```python
from build123d import *
from OCP.BRepFilletAPI import BRepFilletAPI_MakeChamfer

# Parameters (mm, degrees)
SKETCH1_W           = 76.2
SKETCH1_H           = 76.2
SKETCH1_W_2         = 69.85
SKETCH1_H_2         = 69.85
BOSS_EXTRUDE1_DEPTH = 9.525
SKETCH2_R           = 1.26365
CUT_EXTRUDE1_DEPTH  = 86.725
CHAMFER1_SIZE       = 2.54
CHAMFER1_SIZE2      = 2.207988314
SKETCH3_W           = 76.2
SKETCH3_H           = 76.2
SKETCH3_W_2         = 69.85
SKETCH3_H_2         = 69.85
BOSS_EXTRUDE2_DEPTH = 25.4


with BuildPart() as part:
    # Sketch1 → Boss-Extrude1 (new body)
    with BuildSketch(Plane(origin=(0, 0, 0), x_dir=(1, 0, 0), z_dir=(0, 1, 0))):
        Rectangle(SKETCH1_W, SKETCH1_H)
        Rectangle(SKETCH1_W_2, SKETCH1_H_2, mode=Mode.SUBTRACT)
    extrude(amount=BOSS_EXTRUDE1_DEPTH)

    # Sketch2 → Cut-Extrude1 (cut, through all)
    with BuildSketch(Plane.XY.offset(38.1)):
        with Locations((-12.7, 4.7625)):
            Circle(SKETCH2_R)
        with Locations((12.7, 4.7625)):
            Circle(SKETCH2_R)
    extrude(amount=-CUT_EXTRUDE1_DEPTH, mode=Mode.SUBTRACT)

    # Chamfer1: one chamfer whose edges measure the first distance from different faces: ONE call of the kernel's chamfer builder (chamfer() names one face for all edges)
    chamfer1_edges_1 = [part.edges().sort_by_distance(p)[0] for p in [
        (-13.96365, 4.7625, -38.1),
    ]]
    chamfer1_side_1 = [part.faces().sort_by_distance(p)[0] for p in [
        (-13.96365, 4.7625, -36.5125),
    ]]
    chamfer1_edges_2 = [part.edges().sort_by_distance(p)[0] for p in [
        (-13.96365, 4.7625, 38.1),
        (11.43635, 4.7625, 38.1),
    ]]
    chamfer1_side_2 = [part.faces().sort_by_distance(p)[0] for p in [
        (0, 4.7625, 38.1),
    ]]
    chamfer1_edges_3 = [part.edges().sort_by_distance(p)[0] for p in [
        (11.43635, 4.7625, -38.1),
    ]]
    chamfer1_side_3 = [part.faces().sort_by_distance(p)[0] for p in [
        (11.43635, 4.7625, -36.5125),
    ]]
    chamfer1 = BRepFilletAPI_MakeChamfer(part.part.solid().wrapped)
    for e in chamfer1_edges_1:
        chamfer1.Add(CHAMFER1_SIZE, CHAMFER1_SIZE2, e.wrapped, chamfer1_side_1[0].wrapped)  # the first distance lies on this face
    for e in chamfer1_edges_2:
        chamfer1.Add(CHAMFER1_SIZE, CHAMFER1_SIZE2, e.wrapped, chamfer1_side_2[0].wrapped)  # the first distance lies on this face
    for e in chamfer1_edges_3:
        chamfer1.Add(CHAMFER1_SIZE, CHAMFER1_SIZE2, e.wrapped, chamfer1_side_3[0].wrapped)  # the first distance lies on this face
    add(Compound.cast(chamfer1.Shape()), mode=Mode.REPLACE)

    # Sketch3 → Boss-Extrude2 (add)
    with BuildSketch(Plane(origin=(0, 9.525, 0), x_dir=(1, 0, 0), z_dir=(0, 1, 0))):
        Rectangle(SKETCH3_W, SKETCH3_H)
        Rectangle(SKETCH3_W_2, SKETCH3_H_2, mode=Mode.SUBTRACT)
    extrude(amount=BOSS_EXTRUDE2_DEPTH)

    # Mirror2: part across plane


with BuildPart() as part_1:
    add(part.part)
    add(part.part.mirror(Plane.ZX.offset(34.925)))


solid = part_1.part
```
Work out the finished part from the listing and answer in its coordinate system (mm). A direction names the side the tool comes from. Give positions to 0.01 mm unless a question says otherwise; leave off trailing zeros. Order: outer loops, then holes, each group sorted by start corner. A loop starts at its lowest first (then second) coordinate and runs counter-clockwise, first axis right, second up.
1. Section C-C, the plane x = 12.7 is taken. Give the number of separate pieces and of enclosed holes in the cut face, and give its area (3 significant figures).
Result sheet:
separate pieces: 6
enclosed holes: 0
area: 389 mm2
2. Straight lines are drawn through the part: L1, parallel to Y at x = 12.7, z = -35.3; L2, parallel to X at y = 38, z = 26.5 (3 decimals). For each, find the intervals that lie inside material, in ascending order.
Result sheet:
L1: y = 0 to 3.5, 6.03 to 63.82, 66.35 to 69.85
L2: x = -38.1 to -34.925, 34.925 to 38.1
3. Section B-B, the plane y = 51 is taken. Determine the outline of the cut face in (x, z) (3 decimals).
Result sheet:
outline: (-38.1, -38.1) - (38.1, -38.1) - (38.1, 38.1) - (-38.1, 38.1) - close; hole (-34.925, -34.925) - (34.925, -34.925) - (34.925, 34.925) - (-34.925, 34.925) - close
4. Section A-A, the plane x = -3 is taken. Determine the outline of the cut face in (y, z) (3 decimals).
Result sheet:
outline: (0, -38.1) - (69.85, -38.1) - (69.85, -34.925) - (0, -34.925) - close; (0, 34.925) - (69.85, 34.925) - (69.85, 38.1) - (0, 38.1) - close
5. The mould has two halves that part along Z. Classify faces 3 (the flat face through (0, 35, 34.925)), 4 (the flat face through (-1, 35, 38.1)), 5 (the flat face through (-1, 35, -38.1)): released by +Z, released by -Z, zero draft, split by the parting line, or undercut.
Result sheet:
face 3: undercut
face 4: released by +Z
face 5: released by -Z
6. Each of these flat-tipped pins is pushed along its axis until it touches: P1, Ø3, axis at x = 12.7, y = 65.09, coming from the -Z side; P2, Ø3.5, axis at x = -12.7, y = 4.76, coming from the -Z side; P3, Ø4, axis at x = 12.7, y = 65.09, coming from the -Z side. Where does it stop, or does it pass through?
Result sheet:
P1: stops at z = -35.83
P2: stops at z = -36.12
P3: stops at z = -36.41
7. Section D-D, the plane z = -14.5 is taken. Determine the outline of the cut face in (x, y) (3 decimals).
Result sheet:
outline: (-38.1, 0) - (-34.925, 0) - (-34.925, 69.85) - (-38.1, 69.85) - close; (34.925, 0) - (38.1, 0) - (38.1, 69.85) - (34.925, 69.85) - close
8. For faces 1 (the flat face through (-34.925, 35, 0)), 2 (the cylindrical face through (-13.962, 4.818, 35.415)), determine the directions among +Z, -Z, +X, -X, +Y, -Y from which every point of the face is accessible in a straight line to the end or side of a thin tool.
Result sheet:
face 1: +Y, -Y
face 2: +Z, -Z
